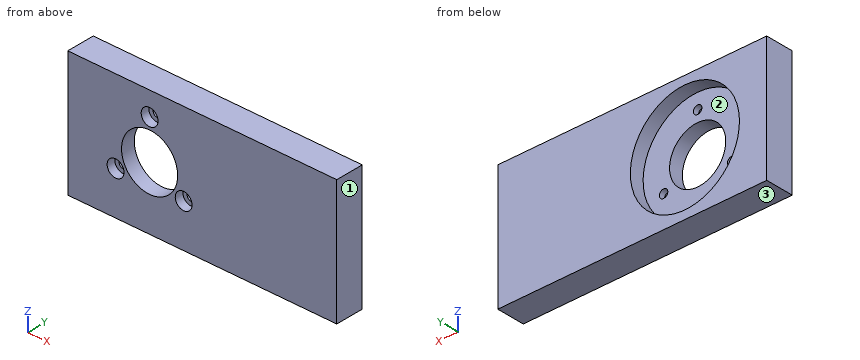
```python
from build123d import *

# Parameters (mm, degrees)
ENCODERSIDEWALLSKETCH_W    = 95.8
ENCODERSIDEWALLSKETCH_H    = 44.8
BOSS_EXTRUDE1_DEPTH        = 10
SKETCH2_R                  = 10
ENCODERAXLECUT_DEPTH       = 10
ENCODERFULLHOLE_R          = 19.425
ENCODERFULLHOLEBORE_DEPTH  = 5
ENCODERSCREWLAYOUTSKETCH_R = 1.5
ENCODERSCREWLAYOUT_DEPTH   = 62.184071257
SKETCH6_R                  = 3
CUT_EXTRUDE4_DEPTH         = 3


with BuildPart() as part:
    # EncoderSideWallSketch → Boss-Extrude1 (new body)
    with BuildSketch(Plane(origin=(0, 0, 0), x_dir=(1, 0, 0), z_dir=(0, 1, 0))):
        with Locations((8.673150268, 0.358937681)):
            Rectangle(ENCODERSIDEWALLSKETCH_W, ENCODERSIDEWALLSKETCH_H)
    extrude(amount=BOSS_EXTRUDE1_DEPTH)

    # Sketch2 → EncoderAxleCut (cut)
    with BuildSketch(Plane(origin=(0, 10, 0), x_dir=(1, 0, 0), z_dir=(0, 1, 0))):
        with Locations(Location((-10.076849732, 0.358937681, 0), (0, 0, 270))):
            Circle(SKETCH2_R)
    extrude(amount=-ENCODERAXLECUT_DEPTH, mode=Mode.SUBTRACT)

    # EncoderFullHole → EncoderFullHoleBore (cut)
    with BuildSketch(Plane(origin=(0, 10, 0), x_dir=(1, 0, 0), z_dir=(0, 1, 0))):
        with Locations(Location((-10.076849732, 0.358937681, 0), (0, 0, 270))):
            Circle(ENCODERFULLHOLE_R)
    extrude(amount=-ENCODERFULLHOLEBORE_DEPTH, mode=Mode.SUBTRACT)

    # EncoderScrewLayoutSketch → EncoderScrewLayout (cut, through all)
    with BuildSketch(Plane(origin=(0, 5, 0), x_dir=(1, 0, 0), z_dir=(0, 1, 0))):
        with Locations(Location((-22.201849732, 7.359309695, 0), (0, 0, 270))):
            Circle(ENCODERSCREWLAYOUTSKETCH_R)
        with Locations(Location((2.048150268, 7.359309695, 0), (0, 0, 270))):
            Circle(ENCODERSCREWLAYOUTSKETCH_R)
        with Locations(Location((-10.076849732, -13.641806347, 0), (0, 0, 270))):
            Circle(ENCODERSCREWLAYOUTSKETCH_R)
    extrude(amount=-ENCODERSCREWLAYOUT_DEPTH, mode=Mode.SUBTRACT)

    # Sketch6 → Cut-Extrude4 (cut)
    with BuildSketch(Plane.XZ):
        with Locations(Location((-10.076849732, 13.641806347, 0), (0, 0, 270))):
            Circle(SKETCH6_R)
        with Locations(Location((-22.201849732, -7.359309695, 0), (0, 0, 270))):
            Circle(SKETCH6_R)
        with Locations(Location((2.048150268, -7.359309695, 0), (0, 0, 270))):
            Circle(SKETCH6_R)
    extrude(amount=-CUT_EXTRUDE4_DEPTH, mode=Mode.SUBTRACT)


solid = part.part
```
Geometry: final body of the model. Coordinates: model frame, mm. Face numbers are marked on the shaded views. Coordinates: 2 decimals unless noted, no trailing zeros. Loops run counter-clockwise (first coordinate to the right, second up) from the corner with the lowest first, then second, coordinate; pieces in that order, holes last. Notation, with made-up numbers: M -5.5,58.5 L 22.5,58.5 A21 cw 22.5,68.5 Z; hole C 10,-19 d2. An arc over 180 degrees is marked long. Put each result on its own line as item: value.
(1) Draft query along X for the marked faces 1, 2 and 3. Return one class per face: pulls with the +X half, pulls with the -X half, needs draft (parallel to the pull), parting line crosses it, or undercut.
Answer sheet:
face 1: pulls with the +X half
face 2: undercut
face 3: needs draft
(2) First-contact query: pin 1 (7 mm diameter, centred on x = 2.05, z = -7.36, fed in from +Y); pin 2 (1.8 mm diameter, centred on x = -22.2, z = -7.36, fed in from -Y); pin 3 (3.5 mm diameter, centred on x = 2.05, z = -7.36, fed in from -Y). Flat tips, straight axial feed; report the tip coordinate or a pass-through.
Answer sheet:
pin 1: stops at y = 5
pin 2: passes through
pin 3: stops at y = 3
(3) Cut plane C-C on z = -3. Return the cut outline in (x, y), then the cut area to 3 significant figures.
Answer sheet:
outline: M -39.23,0 L -19.72,0 L -19.72,5 L -29.32,5 L -29.32,10 L -39.23,10 Z; M -0.43,0 L 56.57,0 L 56.57,10 L 9.17,10 L 9.17,5 L -0.43,5 Z
area: 669 mm^2
(4) Material intervals for probe 1 along Z at (x, y) = (-6, 4.75); probe 2 along Z at (x, y) = (-5, 7.25); probe 3 along Y at (x, z) = (-1, -5), sorted ascending.
Answer sheet:
probe 1: z = -22.76 to -9.49, 8.77 to 22.04
probe 2: z = -22.76 to -19.11, 18.39 to 22.04
probe 3: y = 0 to 5
(5) Cut plane B-B on y = 1. Return the cut outline in (x, z).
Answer sheet:
outline: M -39.23,-22.76 L 56.57,-22.76 L 56.57,22.04 L -39.23,22.04 Z; hole C -22.2,-7.36 d6; hole C -10.08,-0.36 d20; hole C -10.08,13.64 d6; hole C 2.05,-7.36 d6
(6) Cut plane D-D on y = 7. Return the cut outline in (x, z) (3 decimals), then the cut area to 3 significant figures.
Answer sheet:
outline: M -39.227,-22.759 L 56.573,-22.759 L 56.573,22.041 L -39.227,22.041 Z; hole C -10.077,-0.359 d38.85
area: 3,110 mm^2
(7) Cut plane A-A on z = 4. Return the cut outline in (x, y).
Answer sheet:
outline: M -39.23,0 L -19.08,0 L -19.08,5 L -29.01,5 L -29.01,10 L -39.23,10 Z; M -1.08,0 L 56.57,0 L 56.57,10 L 8.85,10 L 8.85,5 L -1.08,5 Z
